The listing builds one solid part. Answer for the finished solid, in the listing's coordinates (mm). Face numbers are marked on the shaded views. A direction names the side the tool comes from. Round coordinates to 2 decimals unless told otherwise and drop trailing zeros. Order: outer loops, then holes, each group sorted by start corner. A loop starts at its lowest first (then second) coordinate and runs counter-clockwise, first axis right, second up. Notation, with made-up numbers: (84.25, 31) - (94.25, 31) arc R27 ccw to (94.25, 66) - close; hole circle Ø9 at (64, 3.25). An arc over 180 degrees is marked (long way). Use CSV: the item, a comma, the result in double quotes. Start each with the question number.
Item 1: Find section A-A, the plane y = 16. Give the vertices of the cut face in (x, z), plus the area to 3 significant figures.
Item 2: Flat-ended cylindrical pins translate along their axes: P1, Ø9, axis at x = 5, y = 45, coming from the -Z side; P2, Ø11, axis at x = -5.5, z = -11, coming from the -Y side; P3, Ø4, axis at y = 47.5, z = -25.5, coming from the +X side. Find the tip coordinate at first contact, or state that the pin passes through.
Item 3: Straight lines are drawn through the part: line 1 along Y through (x, z) = (5, -57.95); line 2 along Y through (x, z) = (5, 1.8); line 3 along Z through (x, y) = (7.75, 41). For each, find the intervals that lie inside material, in ascending order. Write a range as [from, to].
Item 4: For the marked faces 5 and 6, determine the directions among +Z, -Z, +X, -X, +Y, -Y from which every point of the face is accessible in a straight line to the end or side of a thin tool.
Item 5: Find section C-C, the plane z = -56. Count the separate pieces of the cut face and the enclosed holes in it, plus the area to 3 significant figures.
Item 6: Find section B-B, the plane z = -65. Give the vertices of the cut face in (x, y), plus the area to 3 significant figures.
Item 7: Find section D-D, the plane x = -5. Give the vertices of the cut face in (y, z), plus the area to 3 significant figures.
Item 8: Determine the mould class of the marked faces 1, 2, 3 and 4 for opening direction Z: +Z half, -Z half, draft (parallel to the pull), parting line (faces both ways), or undercut.
```python
from build123d import *

# Parameters (mm, degrees)
P_IDAT_VYSUNUT_M1_DEPTH  = 8
SKICA2_R                 = 1.65
ODEBRAT_VYSUNUT_M1_DEPTH = 47.786750261
P_IDAT_VYSUNUT_M2_DEPTH  = 5
SKICA4_R                 = 1.65
ODEBRAT_VYSUNUT_M2_DEPTH = 5
SKICA5_R                 = 1.65
ODEBRAT_VYSUNUT_M3_DEPTH = 55.074023338
ZAOBLIT1_R               = 5
SKICA6_W                 = 2
SKICA6_H                 = 23
P_IDAT_VYSUNUT_M3_DEPTH  = 8
SKICA7_R                 = 2.75
ODEBRAT_VYSUNUT_M4_DEPTH = 2.5
SKICA8_W                 = 10
SKICA8_H                 = 5
P_IDAT_VYSUNUT_M4_DEPTH  = 60
SKICA9_W                 = 8
SKICA9_H                 = 5
P_IDAT_VYSUNUT_M5_DEPTH  = 10
SKICA10_W                = 10
SKICA10_H                = 8
P_IDAT_VYSUNUT_M6_DEPTH  = 45
ZAOBLIT2_R               = 5
SKICA11_R                = 1.65
ODEBRAT_VYSUNUT_M5_DEPTH = 45
ODEBRAT_START            = -2.5
SKICA12_R                = 2.75
ODEBRAT_VYSUNUT_M6_DEPTH = 2.5
SKICA13_R                = 1.65
ODEBRAT_VYSUNUT_M7_DEPTH = 12.5


with BuildPart() as part:
    # Skica1 → Přidat vysunutím1 (new body)
    with BuildSketch(Plane.XY):
        Polygon((0, 0), (10, 0), (10, 10), (8, 10), (8, 33), (10, 33), (10, 45), (0, 45), align=None)
    extrude(amount=P_IDAT_VYSUNUT_M1_DEPTH)

    # Skica2 → Odebrat vysunutím1 (cut, through all)
    with BuildSketch(Plane.XY.offset(8)):
        with Locations((5, 45)):
            Circle(SKICA2_R)
        with Locations((5, 5)):
            Circle(SKICA2_R)
    extrude(amount=-ODEBRAT_VYSUNUT_M1_DEPTH, mode=Mode.SUBTRACT)

    # Skica3 → Přidat vysunutím2 (add)
    with BuildSketch(Plane(origin=(0, 45, 0), x_dir=(1, 0, 0), z_dir=(0, 1, 0))):
        Polygon((0, 0), (0, 10), (-10, 10), (-10, -18), (0, -18), (0, -8), (10, -8), (10, 0), align=None)
    extrude(amount=P_IDAT_VYSUNUT_M2_DEPTH)

    # Skica4 → Odebrat vysunutím2 (cut)
    with BuildSketch(Plane(origin=(0, 50, 0), x_dir=(1, 0, 0), z_dir=(0, 1, 0))):
        with Locations(Location((-5, 5, 0), (0, 0, 270))):
            Circle(SKICA4_R)
        with Locations(Location((-5, -13, 0), (0, 0, 270))):
            Circle(SKICA4_R)
    extrude(amount=-ODEBRAT_VYSUNUT_M2_DEPTH, mode=Mode.SUBTRACT)

    # Skica5 → Odebrat vysunutím3 (cut, through all)
    with BuildSketch(Plane.XY.offset(8)):
        with Locations((5, 45)):
            Circle(SKICA5_R)
    extrude(amount=-ODEBRAT_VYSUNUT_M3_DEPTH, mode=Mode.SUBTRACT)

    # Zaoblit1
    zaoblit1_edges = [part.edges().sort_by_distance(p)[0] for p in [
        (0, 0, 4),
        (10, 0, 4),
        (10, 50, 4),
    ]]
    fillet(zaoblit1_edges, radius=ZAOBLIT1_R - 0.0001)  # a hair under: the kernel refuses the full size

    # Skica6 → Přidat vysunutím3 (add)
    with BuildSketch(Plane.XY.offset(8)):
        with Locations((9, 21.5)):
            Rectangle(SKICA6_W, SKICA6_H)
    extrude(amount=-P_IDAT_VYSUNUT_M3_DEPTH)

    # Skica7 → Odebrat vysunutím4 (cut)
    with BuildSketch(Plane.XY.offset(8)):
        with Locations((5, 5)):
            Circle(SKICA7_R)
        with Locations((5, 45)):
            Circle(SKICA7_R)
    extrude(amount=-ODEBRAT_VYSUNUT_M4_DEPTH, mode=Mode.SUBTRACT)

    # Skica8 → Přidat vysunutím4 (add)
    with BuildSketch(Plane(origin=(0, 0, -10), x_dir=(-1, 0, 0), z_dir=(0, 0, -1))):
        with Locations((5, 47.5)):
            Rectangle(SKICA8_W, SKICA8_H)
    extrude(amount=P_IDAT_VYSUNUT_M4_DEPTH)

    # Skica9 → Přidat vysunutím5 (add)
    with BuildSketch(Plane(origin=(0, 0, 0), x_dir=(0, 0, -1), z_dir=(1, 0, 0))):
        with Locations((56, 47.5)):
            Rectangle(SKICA9_W, SKICA9_H)
    extrude(amount=P_IDAT_VYSUNUT_M5_DEPTH)

    # Skica10 → Přidat vysunutím6 (add)
    with BuildSketch(Plane.XZ.offset(-45)):
        with Locations((5, -56)):
            Rectangle(SKICA10_W, SKICA10_H)
    extrude(amount=P_IDAT_VYSUNUT_M6_DEPTH)

    # Zaoblit2
    zaoblit2_edges = [part.edges().sort_by_distance(p)[0] for p in [
        (10, 50, -56),
        (10, 0, -56),
        (0, 0, -56),
    ]]
    fillet(zaoblit2_edges, radius=ZAOBLIT2_R - 0.0001)  # a hair under: the kernel refuses the full size

    # Skica11 → Odebrat vysunutím5 (cut)
    with BuildSketch(Plane.XY.offset(-52)):
        with Locations((5, 45)):
            Circle(SKICA11_R)
        with Locations((5, 5)):
            Circle(SKICA11_R)
    extrude(amount=-ODEBRAT_VYSUNUT_M5_DEPTH, mode=Mode.SUBTRACT)

    # Skica12 → Odebrat vysunutím6 (cut)
    with BuildSketch(Plane(origin=(0, 0, -60), x_dir=(-1, 0, 0), z_dir=(0, 0, -1)).offset(ODEBRAT_START)):
        with Locations(Location((-5, 45, 0), (0, 0, 180))):
            Circle(SKICA12_R)
        with Locations(Location((-5, 5, 0), (0, 0, 180))):
            Circle(SKICA12_R)
    extrude(amount=ODEBRAT_VYSUNUT_M6_DEPTH, mode=Mode.SUBTRACT)

    # Skica13 → Odebrat vysunutím7 (cut)
    with BuildSketch(Plane(origin=(0, 50, 0), x_dir=(1, 0, 0), z_dir=(0, 1, 0))):
        with Locations(Location((-5, 65, 0), (0, 0, 270))):
            Circle(SKICA13_R)
        with Locations(Location((-5, 47, 0), (0, 0, 270))):
            Circle(SKICA13_R)
    extrude(amount=-ODEBRAT_VYSUNUT_M7_DEPTH, mode=Mode.SUBTRACT)


solid = part.part
```
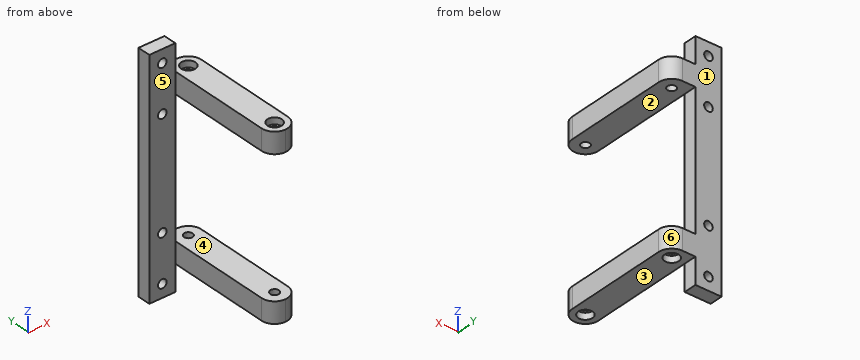
Worked out:
1,outline,"(0, -60) - (10, -60) - (10, -52) - (0, -52) - close; (0, 0) - (10, 0) - (10, 8) - (0, 8) - close"
1,area,"160 mm²"
2,P1,"stops at z = -60"
2,P2,"stops at y = 45"
2,P3,"stops at x = 0"
3,line 1,"y = [0, 2.25], [7.75, 42.25], [47.75, 50]"
3,line 2,"y = [0, 3.35], [6.65, 43.35], [46.65, 50]"
3,line 3,"z = [-60, -52], [0, 8]"
4,face 5,"+Z, -Z, -X, -Y"
4,face 6,"+Z, -Z, +X, +Y"
5,separate pieces,"1"
5,enclosed holes,"2"
5,area,"517 mm²"
6,outline,"(-10, 45) - (-6.65, 45) - (-6.65, 50) - (-10, 50) - close; (-3.35, 45) - (0, 45) - (0, 50) - (-3.35, 50) - close"
6,area,"33.5 mm²"
7,outline,"(45, -70) - (50, -70) - (50, -66.65) - (45, -66.65) - close; (45, -63.35) - (50, -63.35) - (50, -48.65) - (45, -48.65) - close; (45, -45.35) - (50, -45.35) - (50, -6.65) - (45, -6.65) - close; (45, -3.35) - (50, -3.35) - (50, 11.35) - (45, 11.35) - close; (45, 14.65) - (50, 14.65) - (50, 18) - (45, 18) - close"
7,area,"374 mm²"
8,face 1,"draft"
8,face 2,"undercut"
8,face 3,"-Z half"
8,face 4,"undercut"
